Design review of the part shown in the three views and the two pictorial views. Dimensions are in mm from the part's minimum x, y and z. A direction names the side the tool comes from. Coordinates: 2 decimals unless noted, no trailing zeros. Loops run counter-clockwise (first coordinate to the right, second up) from the corner with the lowest first, then second, coordinate; pieces in that order, holes last. Notation, with made-up numbers: (5.25, 21.5) -> (53.25, 21.5) arc R29 ccw to (53.25, 55.5) -> close; hole circle Ø4 at (70, 40). An arc over 180 degrees is marked (long way). One line per item, written item: value.
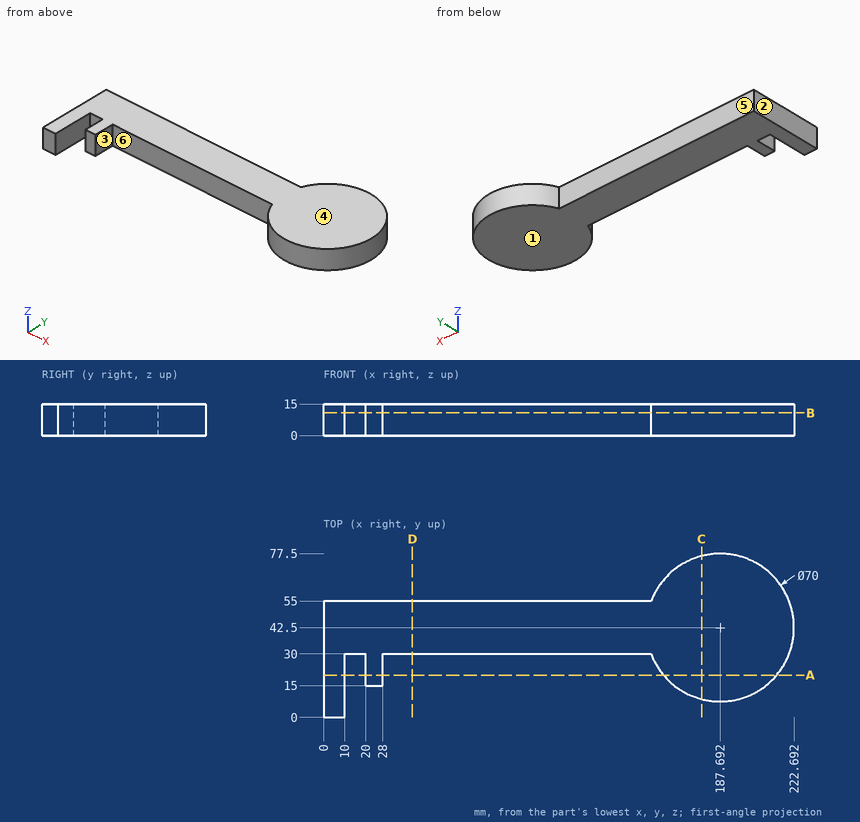
1. Take a section at C-C, the plane x = 179. Give the boundary of the cut face in (y, z).
Return value:
outline: (8.6, 0) -> (76.4, 0) -> (76.4, 15) -> (8.6, 15) -> close
2. Take a section at B-B, the plane z = 10.75. Give the boundary of the cut face in (x, y).
Return value:
outline: (0, 0) -> (10, 0) -> (10, 30) -> (20, 30) -> (20, 15) -> (28, 15) -> (28, 30) -> (155, 30) arc R35 ccw (long way) to (155, 55) -> (0, 55) -> close
3. To check wall thickness, follow probe 1 along X at (y, z) = (17, 11.25) (1 decimal); probe 2 along Y at (x, z) = (91, 3.5); probe 3 along X at (y, z) = (24.5, 1.75) (1 decimal). State the ranges of each line that lie inside material, in increasing order. Write a range as from..to.
Return value:
probe 1: x = 0..10, 20..28, 163.7..211.7
probe 2: y = 30..55
probe 3: x = 0..10, 20..28, 157.7..217.7
4. For the marked faces 4, 5 and 6, list the 3-axis set-ups (+Z, -Z, +X, -X, +Y, -Y) from which the entire face can be reached by the end or side of a thin tool; tool diameter is ignored.
Return value:
face 4: +Z, +X, -X, +Y, -Y
face 5: +Z, -Z, -X, +Y
face 6: +Z, -Z, -Y
5. Take a section at A-A, the plane y = 20. Give the boundary of the cut face in (x, z).
Return value:
outline: (0, 0) -> (10, 0) -> (10, 15) -> (0, 15) -> close; (20, 0) -> (28, 0) -> (28, 15) -> (20, 15) -> close; (160.88, 0) -> (214.5, 0) -> (214.5, 15) -> (160.88, 15) -> close
6. The part is to be moulded in two halves that separate along X. For the marked faces 1, 2 and 3, say which applies: pulls with the +X half, pulls with the -X half, needs draft (parallel to the pull), parting line crosses it, or undercut.
Return value:
face 1: needs draft
face 2: pulls with the -X half
face 3: undercut
7. Take a section at D-D, the plane x = 42. Give the boundary of the cut face in (y, z).
Return value:
outline: (30, 0) -> (55, 0) -> (55, 15) -> (30, 15) -> close
8. Insertion check: pin 1 Ø7.5 at (y, z) = (12, 10.5) entering from +X; pin 2 Ø5 at (x, z) = (116.5, 9) entering from +Y; pin 3 Ø3 at (y, z) = (9, 3) entering from +X. Each pin has a flat end and moves straight along its axis. Give the tip position at first contact, or say it passes through.
Return value:
pin 1: stops at x = 210.26
pin 2: stops at y = 55
pin 3: stops at x = 201.87
